Solid Edge part; units mm, degrees
sketch "Sketch1" plane through (28, 0, 0) normal (1, 0, 0) x (0, 1, 0)
  line L0 (-256.284, 13.8) -> (-206.284, 13.8)
  line L1 (-206.284, 13.8) -> (-206.284, 13)
  line L2 (-256.284, 13) -> (-206.284, 13)
  line L3 (-256.284, 13) -> (-256.284, 13.8)
extrude "Protrusion1" add sketch "Sketch1" against normal blind 18
sketch "Sketch2" plane through (19, -249.0202, 13.8) normal (0, 0, 1) x (0, 1, 0)
  line L0 (4.7362, 9) -> (4.7362, -1)
  line L1 (4.7362, -1) -> (44.7362, -1)
  line L2 (44.7362, -1) -> (44.7362, 9)
  line L3 (44.7362, 9) -> (4.7362, 9)
  circle A0 centre (-1.2638, 3) radius 2.2
  dimension "D1" = 44.7362
  dimension "D2" = 44.7362
extrude "Cutout1" cut sketch "Sketch2" along normal through all and the other way through all
sketch "Sketch3" plane through (19, -231.284, 13) normal (0, 0, -1) x (1, 0, 0)
  line L0 (1, 8) -> (9, 8)
  line L1 (9, -4) -> (9, 8)
  line L2 (9, -4) -> (1, -4)
  line L3 (1, 8) -> (1, -4)
  dimension "D1" = 1
extrude "ExtrudedCutout_4" cut sketch "Sketch3" against normal blind 0.1
Source: CAD feature listing. Evaluate the final solid. Frame: model axes, mm. A direction names the side the tool comes from. Round coordinates to 2 decimals unless told otherwise and drop trailing zeros. Loops run counter-clockwise (first coordinate to the right, second up) from the corner with the lowest first, then second, coordinate; pieces in that order, holes last. Notation, with made-up numbers: M 28,44.5 L 85,44.5 A17 cw 85,77.5 Z; hole C 19,81.25 d5. An arc over 180 degrees is marked long. Use a Markdown table: item, result. Add a question column.
1. Reachability of faces 1 (the flat face through (20, -225.6, 13.4)), 2 (the flat face through (19.1, -256.284, 13.4)) from +Z, -Z, +X, -X, +Y, -Y: full face, straight path, thin tool, end or side. Return the list, or none.
2. Contact query for a flat-ended pin moving along its axis: P1, Ø2.5, axis at x = 16, y = -250.284, coming from the -Z side. Output: stop coordinate, or through.
3. Section query C-C on x = 27. Return the cut outline in (y, z).
4. Section query D-D on y = -251. Return the cut outline in (x, z).
5. Section query B-B on x = 16. Return the cut outline in (y, z), then the cut area to 3 significant figures.
6. Mould query, pull axis Y, two halves, no side actions, for faces 3 (the cylindrical face through (15.9, -252.48, 13.41)), 4 (the flat face through (24, -217, 13)), 5 (the flat face through (24, -233, 13.1)), 6 (the flat face through (24.1, -206.284, 13.4)). Classes: pulls with the +Y half, pulls with the -Y half, needs draft (parallel to the pull), parting line crosses it, or undercut.
7. Section query A-A on z = 13.3. Return the cut outline in (x, y), then the cut area to 3 significant figures.
8. Line query: line 1 (Y direction, x = 16, z = 13.55); line 2 (X direction, y = -226.5, z = 13.45); line 3 (Y direction, x = 14.25, z = 13.7). Output: solid intervals per line, ascending.
Reported:
| question | item | result |
|---|---|---|
| 1 | face 1 | +Z, -Z, -X, +Y |
| 1 | face 2 | +Z, -Z, +X, -X, -Y |
| 2 | P1 | passes through |
| 3 | outline | M -256.28,13 L -239.28,13 L -239.28,13.1 L -227.28,13.1 L -227.28,13 L -206.28,13 L -206.28,13.8 L -256.28,13.8 Z |
| 4 | outline | M 10,13 L 13.92,13 L 13.92,13.8 L 10,13.8 Z; M 18.08,13 L 28,13 L 28,13.8 L 18.08,13.8 Z |
| 5 | outline | M -256.28,13 L -252.48,13 L -252.48,13.8 L -256.28,13.8 Z; M -248.08,13 L -244.28,13 L -244.28,13.8 L -248.08,13.8 Z |
| 5 | area | 6.08 mm² |
| 6 | face 3 | undercut |
| 6 | face 4 | needs draft |
| 6 | face 5 | undercut |
| 6 | face 6 | pulls with the +Y half |
| 7 | outline | M 10,-256.28 L 28,-256.28 L 28,-206.28 L 20,-206.28 L 20,-244.28 L 10,-244.28 Z; hole C 16,-250.28 d4.4 |
| 7 | area | 505 mm² |
| 8 | line 1 | y = -256.28 to -252.48, -248.08 to -244.28 |
| 8 | line 2 | x = 20 to 28 |
| 8 | line 3 | y = -256.28 to -251.62, -248.95 to -244.28 |
